Drawing for the job (mm, zero at the part's lowest x, y, z). A direction names the side the tool comes from. Coordinates: 2 decimals unless noted, no trailing zeros. Write each loop counter-clockwise with the first axis right and the second up, starting at its lowest first coordinate (ties: lowest second). Pieces come first, ordered by that corner, then holes. Notation, with made-up numbers: (-20, 44) - (-11, 44) arc R10 cw to (-11, 54) - close; hole circle Ø4 at (8, 68.25). An arc over 180 degrees is marked (long way). Write each question's results on one line, items separated by ' | '.
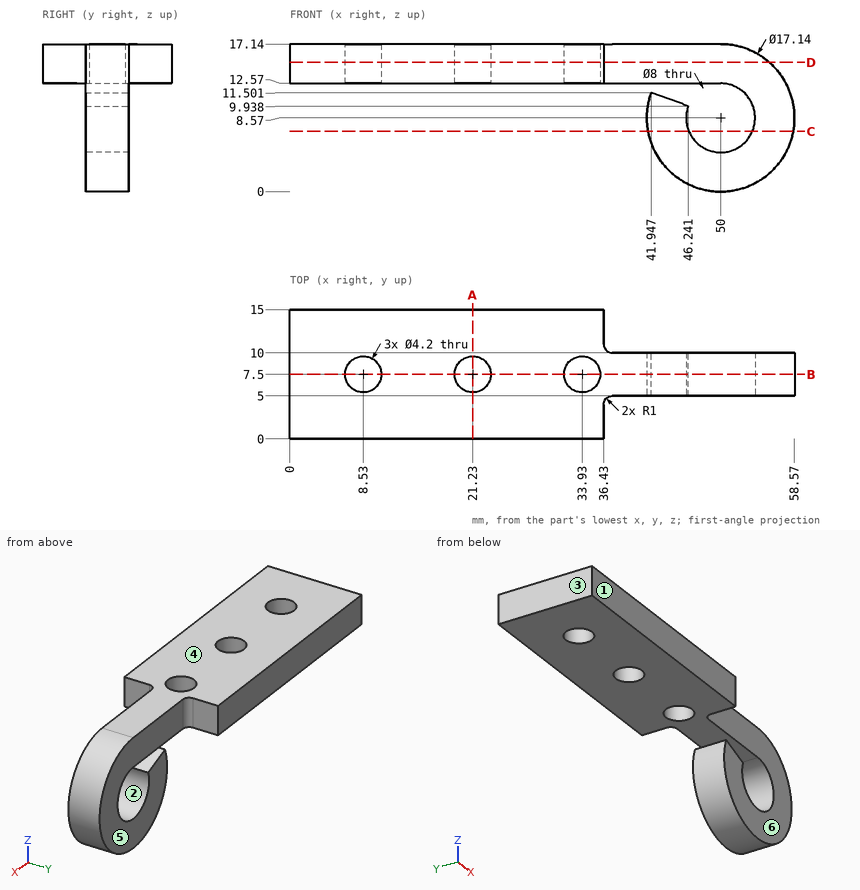
(1) 3-axis set-ups, long thin cutter, end or side, ignore diameter. For the marked faces 4, 5 and 6: which of +Z, -Z, +X, -X, +Y, -Y reach the whole face in a straight line?
Return value:
face 4: +Z, +X, -X, +Y, -Y | face 5: +Z, -Z, +X, +Y | face 6: +Z, -Z, +X, -Y
(2) Saw through at D-D on z = 15. Write the cut outline in (x, y).
Return value:
outline: (0, 0) - (36.43, 0) - (36.43, 4) arc R1 cw to (37.43, 5) - (55.67, 5) - (55.67, 10) - (37.43, 10) arc R1 cw to (36.43, 11) - (36.43, 15) - (0, 15) - close; hole circle Ø4.2 at (8.53, 7.5); hole circle Ø4.2 at (21.23, 7.5); hole circle Ø4.2 at (33.93, 7.5)
(3) Two-plate mould, pull along X, no slides. Class the marked faces 1, 2 and 3: released by +X, released by -X, zero draft, split by the parting line, or undercut.
Return value:
face 1: zero draft | face 2: undercut | face 3: released by -X
(4) Saw through at A-A on x = 21.23. Write the cut outline in (y, z).
Return value:
outline: (0, 12.57) - (5.4, 12.57) - (5.4, 17.14) - (0, 17.14) - close; (9.6, 12.57) - (15, 12.57) - (15, 17.14) - (9.6, 17.14) - close
(5) Saw through at C-C on z = 7. Write the cut outline in (x, y) (1 decimal).
Return value:
outline: (41.6, 5) - (46.3, 5) - (46.3, 10) - (41.6, 10) - close; (53.7, 5) - (58.4, 5) - (58.4, 10) - (53.7, 10) - close
(6) Flat gauge pins, fed straight in: P1, Ø8, axis at x = 7, y = 3.5, coming from the -Z side; P2, Ø4.5, axis at y = 13.5, z = 14, coming from the +X side. Where does each tip first touch, or does it go through?
Return value:
P1: stops at z = 12.57 | P2: stops at x = 36.43
(7) Wall check: line 1 (X direction, y = 8.6, z = 8.57); line 2 (Y direction, x = 21.23, z = 15.5); line 3 (Z direction, x = 50, y = 8.95). Give the ranges that are in metal, low to high. Write a range as from..to.
Return value:
line 1: x = 41.43..46, 54..58.57 | line 2: y = 0..5.4, 9.6..15 | line 3: z = 0..4.57, 12.57..17.14
(8) Saw through at B-B on y = 7.5. Write the cut outline in (x, z).
Return value:
outline: (0, 12.57) - (6.43, 12.57) - (6.43, 17.14) - (0, 17.14) - close; (10.63, 12.57) - (19.13, 12.57) - (19.13, 17.14) - (10.63, 17.14) - close; (23.33, 12.57) - (31.83, 12.57) - (31.83, 17.14) - (23.33, 17.14) - close; (36.03, 12.57) - (50, 12.57) arc R4 cw (long way) to (46.24, 9.94) - (41.95, 11.5) arc R8.57 ccw (long way) to (50, 17.14) - (36.03, 17.14) - close
